Design review of the part shown in the three views and the two pictorial views. Dimensions are in mm from the part's minimum x, y and z. A direction names the side the tool comes from. Coordinates: 2 decimals unless noted, no trailing zeros. Write each loop counter-clockwise with the first axis right and the second up, starting at its lowest first coordinate (ties: lowest second). Pieces come first, ordered by that corner, then holes. Notation, with made-up numbers: (40.25, 75) - (51.25, 75) arc R32 ccw to (51.25, 105) - close; hole circle Ø6 at (-26.75, 15.5). An arc over 180 degrees is marked (long way). Answer as CSV lines item,"result". Start each with the question number.
Q1. We need section B-B (z = 19.5). Write out the cut boundary in (x, y), plus the area to 3 significant figures.
Q2. For line 1 along X through (y, z) = (4.5, 29); line 2 along Y through (x, z) = (36.5, 11.5); line 3 along Z through (x, y) = (7.5, 12), list the stretches that pass through material, from the lowest coordinate up. Write a range as [from, to].
Q3. We need section D-D (z = 49). Write out the cut boundary in (x, y), plus the area to 3 significant figures.
Q4. We need section C-C (y = 16.5). Write out the cut boundary in (x, z), plus the area to 3 significant figures.
Q5. Clearance check with flat-ended pins moving along their axes: pin 1 (5 mm diameter, centred on x = 36.5, y = 36.5, fed in from +Z); pin 2 (5 mm diameter, centred on x = 27.5, y = 27, fed in from +Z); pin 3 (12 mm diameter, centred on y = 28, z = 47.5, fed in from -X). State where each tip first meets the part, or that it passes through.
Q6. Machinability: for the marked faces 1 and 2, which of the approach directions +Z, -Z, +X, -X, +Y, -Y give a long, thin tool a straight path to every point of the face, cutting with its end or side? Answer none if there is none.
Q7. We need section A-A (x = 21). Write out the cut boundary in (y, z).
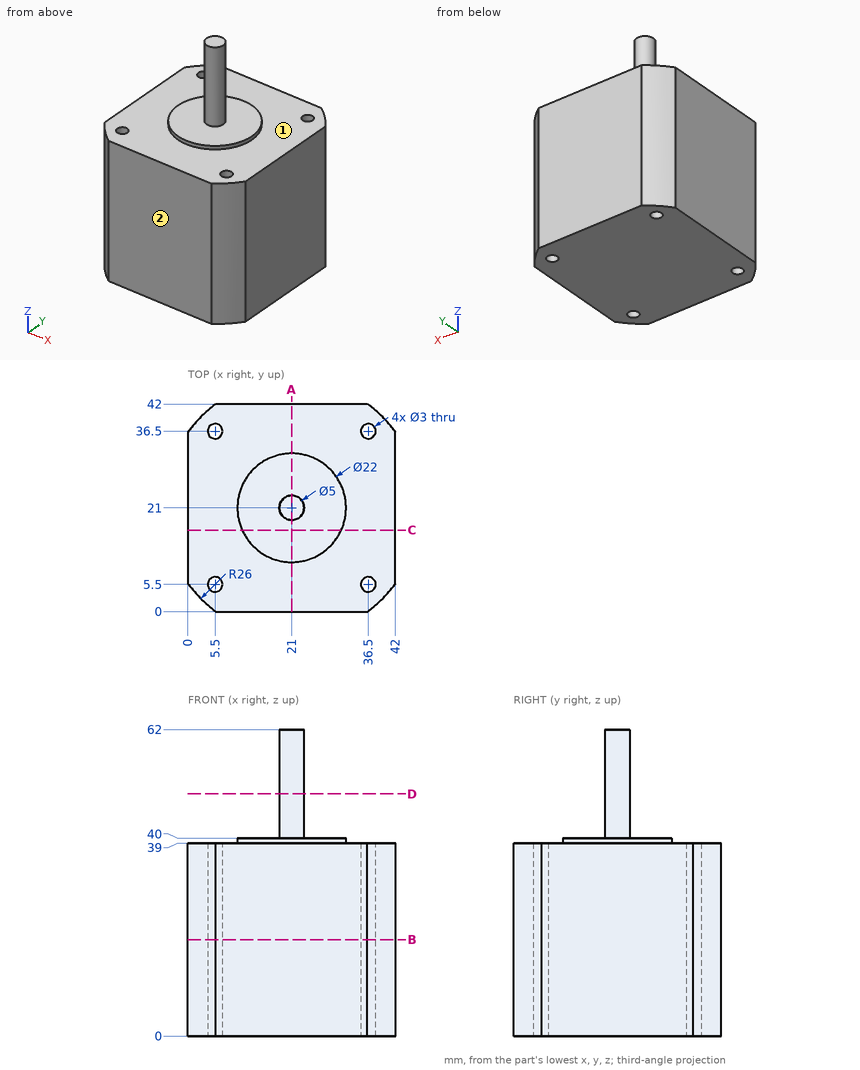
Results list:
1,outline,"(0, 5.67) arc R26 ccw to (5.67, 0) - (36.33, 0) arc R26 ccw to (42, 5.67) - (42, 36.33) arc R26 ccw to (36.33, 42) - (5.67, 42) arc R26 ccw to (0, 36.33) - close; hole circle Ø3 at (5.5, 5.5); hole circle Ø3 at (5.5, 36.5); hole circle Ø3 at (36.5, 5.5); hole circle Ø3 at (36.5, 36.5)"
1,area,"1,680 mm2"
2,line 1,"x = [0.91, 4.38], [6.62, 35.38], [37.62, 41.09]"
2,line 2,"y = [0.13, 4], [7, 35], [38, 41.87]"
2,line 3,"z = [0, 39]"
3,outline,"circle Ø5 at (21, 21)"
3,area,"19.6 mm2"
4,outline,"(0, 0) - (42, 0) - (42, 39) - (31.04, 39) - (31.04, 40) - (10.96, 40) - (10.96, 39) - (0, 39) - close"
4,area,"1,660 mm2"
5,pin 1,"stops at z = 39"
5,pin 2,"stops at z = 40"
5,pin 3,"stops at x = 18.71"
6,face 1,"+Z"
6,face 2,"+Z, -Z, +X, -X, -Y"
7,outline,"(0, 0) - (42, 0) - (42, 39) - (32, 39) - (32, 40) - (23.5, 40) - (23.5, 62) - (18.5, 62) - (18.5, 40) - (10, 40) - (10, 39) - (0, 39) - close"
